Study the drawing (mm; zero at the part's minimum x, y, z) and answer. Coordinates: 2 decimals unless noted, no trailing zeros. Loops run counter-clockwise (first coordinate to the right, second up) from the corner with the lowest first, then second, coordinate; pieces in that order, holes last. Notation, with made-up numbers: (-17, 53.25) - (18, 53.25) arc R14 ccw to (18, 63.25) - close; hole circle Ø6 at (85.25, 11). An arc over 180 degrees is marked (long way). Write each question's results on one line, items separated by ' | '. Start each with the question number.
(1) Find section A-A on z = 0.4. Determine the outline of the cut face in (x, y).
(2) Find section B-B on x = 36.5. Determine the outline of the cut face in (y, z).
(3) Consider line 1 (X direction, y = 3, z = 3.7); line 2 (X direction, y = 3.5, z = 4.5); line 3 (Y direction, x = 36.5, z = 4). Determine where each line is inside the solid, lowest interval first. Write a range as from..to.
(4) Given pin 1 Ø3 at (y, z) = (8, 0.5) entering from -X; pin 2 Ø1 at (y, z) = (11, 4) entering from +X, each flat-ended and moving along its own axis, determine where each tip first touches the part or whether it passes through.
(5) Find section C-C on y = 12.25. Determine the outline of the cut face in (x, z).
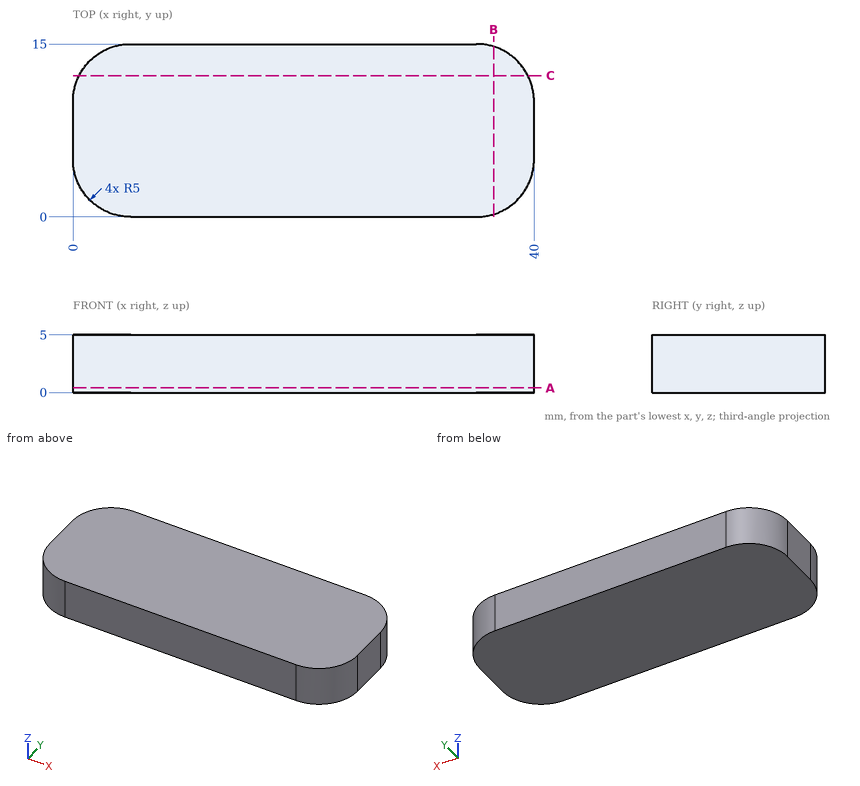
Values:
1) outline: (0, 5) arc R5 ccw to (5, 0) - (35, 0) arc R5 ccw to (40, 5) - (40, 10) arc R5 ccw to (35, 15) - (5, 15) arc R5 ccw to (0, 10) - close
2) outline: (0.23, 0) - (14.77, 0) - (14.77, 5) - (0.23, 5) - close
3) line 1: x = 0.42..39.58 | line 2: x = 0.23..39.77 | line 3: y = 0.23..14.77
4) pin 1: stops at x = 0 | pin 2: stops at x = 39.97
5) outline: (0.53, 0) - (39.47, 0) - (39.47, 5) - (0.53, 5) - close
